```python
from build123d import *

# Parameters (mm, degrees)
F1_DEPTH = 63.7
F2_R     = 1.5
F3_DEPTH = 25
F4_DEPTH = 8


with BuildPart() as f1:
    # F0 (on Front) → F1 (new body)
    with BuildSketch(Plane.XZ):
        Polygon((0, 25), (0, 0), (6, 0), (6, 10), (9, 10), (9, 0), (15, 0), (15, 25), (12, 25), (12, 15), (3, 15), (3, 25), align=None)
    extrude(amount=-F1_DEPTH)

    # F2 (on face) → F3 (cut)
    with BuildSketch(Plane.YZ.offset(15)):
        with Locations((31.85, 20)):
            Circle(F2_R)
    extrude(amount=-F3_DEPTH, mode=Mode.SUBTRACT)

    # F2 (on face) → F4 (cut)
    with BuildSketch(Plane.YZ.offset(15)):
        with Locations((31.85, 4)):
            Circle(F2_R)
    extrude(amount=-F4_DEPTH, mode=Mode.SUBTRACT)


solid = f1.part
```
Check sheet for the modelled part. Datum: model origin and axes. Units: mm. A direction names the side the tool comes from. Round coordinates to 2 decimals unless told otherwise and drop trailing zeros. Order: outer loops, then holes, each group sorted by start corner. A loop starts at its lowest first (then second) coordinate and runs counter-clockwise, first axis right, second up.
1) Section check A-A (z = 20). Record the boundary of the cut face in (x, y).
2) Tool access check on faces 1 (the flat face through (12, 31, 22)), 2 (the cylindrical face through (12.04, 30.35, 4.07)), 3 (the flat face through (7, 31, 10)), 4 (the flat face through (5.7, 63.7, 9.9)). Record the directions out of +Z, -Z, +X, -X, +Y, -Y that give a thin tool (end or side, any length) a straight path to the whole face; none if there is none.
3) Go/stop test with flat-tipped pins: pin 1 Ø2.5 at (x, y) = (6.5, 22) entering from +Z; pin 2 Ø2.5 at (y, z) = (31.85, 20) entering from -X. Record where each tip stops, or that it passes through.
4) Section check B-B (y = 31.85). Record the boundary of the cut face in (x, z).
5) Section check C-C (z = 22.75). Record the boundary of the cut face in (x, y).
6) Mould release check, pull along X, two halves, no side actions. Record for faces 5 (the flat face through (15, 31, 12)), 6 (the flat face through (6, 31, 5)), 7 (the flat face through (0, 31, 13)), 8 (the cylindrical face through (1.52, 30.35, 20.07)): +X half, -X half, draft (parallel to the pull), parting line (faces both ways), or undercut.
7) Section check D-D (z = 4). Record the boundary of the cut face in (x, y), and give its area (3 significant figures).
8) Scan lines: line 1 (Z direction, x = 13.15, y = 31.85); line 2 (X direction, y = 34, z = 19); line 3 (X direction, y = 54.5, z = 6.75). Record each from-to range of solid material in increasing order.
Result:
1. outline: (0, 0) - (3, 0) - (3, 30.35) - (0, 30.35) - close; (0, 33.35) - (3, 33.35) - (3, 63.7) - (0, 63.7) - close; (12, 0) - (15, 0) - (15, 30.35) - (12, 30.35) - close; (12, 33.35) - (15, 33.35) - (15, 63.7) - (12, 63.7) - close
2. face 1: +Z, +Y, -Y
2. face 2: +X
2. face 3: -Z, +Y, -Y
2. face 4: +Z, -Z, +X, -X, +Y
3. pin 1: stops at z = 15
3. pin 2: passes through
4. outline: (0, 0) - (6, 0) - (6, 10) - (9, 10) - (9, 5.5) - (15, 5.5) - (15, 18.5) - (12, 18.5) - (12, 15) - (3, 15) - (3, 18.5) - (0, 18.5) - close; (0, 21.5) - (3, 21.5) - (3, 25) - (0, 25) - close; (9, 0) - (15, 0) - (15, 2.5) - (9, 2.5) - close; (12, 21.5) - (15, 21.5) - (15, 25) - (12, 25) - close
5. outline: (0, 0) - (3, 0) - (3, 63.7) - (0, 63.7) - close; (12, 0) - (15, 0) - (15, 63.7) - (12, 63.7) - close
6. face 5: +X half
6. face 6: undercut
6. face 7: -X half
6. face 8: draft
7. outline: (0, 0) - (6, 0) - (6, 63.7) - (0, 63.7) - close; (9, 0) - (15, 0) - (15, 30.35) - (9, 30.35) - close; (9, 33.35) - (15, 33.35) - (15, 63.7) - (9, 63.7) - close
7. area: 746 mm2
8. line 1: z = 0 to 2.5, 5.5 to 18.5, 21.5 to 25
8. line 2: x = 0 to 3, 12 to 15
8. line 3: x = 0 to 6, 9 to 15
